Geometry check sheet. Reference: the model listing, model coordinates, mm. Give positions to 0.01 mm unless a question says otherwise; leave off trailing zeros. Loops run counter-clockwise (first coordinate to the right, second up) from the corner with the lowest first, then second, coordinate; pieces in that order, holes last.
1. Cross-section at B-B, the plane x = 42.5. Record the cut outline in (y, z), plus the area to 3 significant figures.
2. Go/stop test with flat-tipped pins: pin 1 Ø1.5 at (x, y) = (-1, 1.5) entering from -Z; pin 2 Ø1.5 at (y, z) = (2.5, -117) entering from +X; pin 3 Ø1.5 at (y, z) = (2.5, -71.5) entering from -X. Record where each tip stops, or that it passes through.
3. Material ranges on L1, parallel to X at y = 0.85, z = -80; L2, parallel to Z at x = 105, y = 2.75, recorded low to high.
4. Cross-section at A-A, the plane z = -87. Record the cut outline in (x, y).
from build123d import *

# Parameters (mm, degrees)
SKETCH1_W            = 150
SKETCH1_H            = 150
BOSS_EXTRUDE9_DEPTH  = 3
SKETCH8_W            = 20
SKETCH8_H            = 3
BOSS_EXTRUDE10_DEPTH = 3
SKETCH9_W            = 20
SKETCH9_H            = 3
BOSS_EXTRUDE11_DEPTH = 3
SKETCH10_W           = 20
SKETCH10_H           = 3
BOSS_EXTRUDE12_DEPTH = 3
SKETCH11_W           = 20
SKETCH11_H           = 3
BOSS_EXTRUDE13_DEPTH = 3
SKETCH13_W           = 20
SKETCH13_H           = 3
BOSS_EXTRUDE14_DEPTH = 3
SKETCH14_W           = 20
SKETCH14_H           = 3
BOSS_EXTRUDE15_DEPTH = 3
SKETCH15_W           = 20
SKETCH15_H           = 3
BOSS_EXTRUDE16_DEPTH = 3
SKETCH16_W           = 20
SKETCH16_H           = 3
BOSS_EXTRUDE17_DEPTH = 3


with BuildPart() as part:
    # Sketch1 → Boss-Extrude9 (new body)
    with BuildSketch(Plane(origin=(0, 0, 0), x_dir=(1, 0, 0), z_dir=(0, 1, 0))):
        with Locations((75, 75)):
            Rectangle(SKETCH1_W, SKETCH1_H)
    extrude(amount=BOSS_EXTRUDE9_DEPTH)

    # Sketch8 → Boss-Extrude10 (add)
    with BuildSketch(Plane.ZY):
        with Locations((-20, 1.5)):
            Rectangle(SKETCH8_W, SKETCH8_H)
    extrude(amount=BOSS_EXTRUDE10_DEPTH)

    # Sketch9 → Boss-Extrude11 (add)
    with BuildSketch(Plane.XY):
        with Locations((20, 1.5)):
            Rectangle(SKETCH9_W, SKETCH9_H)
    extrude(amount=BOSS_EXTRUDE11_DEPTH)

    # Sketch10 → Boss-Extrude12 (add)
    with BuildSketch(Plane.XY):
        with Locations((130, 1.5)):
            Rectangle(SKETCH10_W, SKETCH10_H)
    extrude(amount=BOSS_EXTRUDE12_DEPTH)

    # Sketch11 → Boss-Extrude13 (add)
    with BuildSketch(Plane(origin=(150, 0, 0), x_dir=(0, 0, -1), z_dir=(1, 0, 0))):
        with Locations((20, 1.5)):
            Rectangle(SKETCH11_W, SKETCH11_H)
    extrude(amount=BOSS_EXTRUDE13_DEPTH)

    # Sketch13 → Boss-Extrude14 (add)
    with BuildSketch(Plane(origin=(150, 0, 0), x_dir=(0, 0, -1), z_dir=(1, 0, 0))):
        with Locations((130, 1.5)):
            Rectangle(SKETCH13_W, SKETCH13_H)
    extrude(amount=BOSS_EXTRUDE14_DEPTH)

    # Sketch14 → Boss-Extrude15 (add)
    with BuildSketch(Plane(origin=(0, 0, -150), x_dir=(-1, 0, 0), z_dir=(0, 0, -1))):
        with Locations((-130, 1.5)):
            Rectangle(SKETCH14_W, SKETCH14_H)
    extrude(amount=BOSS_EXTRUDE15_DEPTH)

    # Sketch15 → Boss-Extrude16 (add)
    with BuildSketch(Plane(origin=(0, 0, -150), x_dir=(-1, 0, 0), z_dir=(0, 0, -1))):
        with Locations((-20, 1.5)):
            Rectangle(SKETCH15_W, SKETCH15_H)
    extrude(amount=BOSS_EXTRUDE16_DEPTH)

    # Sketch16 → Boss-Extrude17 (add)
    with BuildSketch(Plane.ZY):
        with Locations((-130, 1.5)):
            Rectangle(SKETCH16_W, SKETCH16_H)
    extrude(amount=BOSS_EXTRUDE17_DEPTH)


solid = part.part
Result:
1. outline: (0, -150) - (3, -150) - (3, 0) - (0, 0) - close
1. area: 450 mm2
2. pin 1: stops at z = -140
2. pin 2: stops at x = 150
2. pin 3: stops at x = 0
3. L1: x = 0 to 150
3. L2: z = -150 to 0
4. outline: (0, 0) - (150, 0) - (150, 3) - (0, 3) - close
